from build123d import *

# Parameters (mm, degrees)
SKETCH1_W           = 145
SKETCH1_H           = 67
SKETCH1_R           = 1.5
BOSS_EXTRUDE1_DEPTH = 3.175
FILLET2_R           = 2


with BuildPart() as part:
    # Sketch1 → Boss-Extrude1 (new body)
    with BuildSketch(Plane.XY):
        Rectangle(SKETCH1_W, SKETCH1_H)
        with Locations((-35, 23.5)):
            Circle(SKETCH1_R, mode=Mode.SUBTRACT)
        with Locations((35, 23.5)):
            Circle(SKETCH1_R, mode=Mode.SUBTRACT)
        with Locations((35, -23.5)):
            Circle(SKETCH1_R, mode=Mode.SUBTRACT)
        with Locations((-35, -23.5)):
            Circle(SKETCH1_R, mode=Mode.SUBTRACT)
        with Locations((-27.5, 15)):
            Circle(SKETCH1_R, mode=Mode.SUBTRACT)
        with Locations((27.5, 15)):
            Circle(SKETCH1_R, mode=Mode.SUBTRACT)
        with Locations((27.5, -15)):
            Circle(SKETCH1_R, mode=Mode.SUBTRACT)
        with Locations((-27.5, -15)):
            Circle(SKETCH1_R, mode=Mode.SUBTRACT)
        with Locations((-69, 30)):
            Circle(SKETCH1_R, mode=Mode.SUBTRACT)
        with Locations((-50, 30)):
            Circle(SKETCH1_R, mode=Mode.SUBTRACT)
        with Locations((-50, -30)):
            Circle(SKETCH1_R, mode=Mode.SUBTRACT)
        with Locations((-69, -30)):
            Circle(SKETCH1_R, mode=Mode.SUBTRACT)
        with Locations((50, -30)):
            Circle(SKETCH1_R, mode=Mode.SUBTRACT)
        with Locations((69, -30)):
            Circle(SKETCH1_R, mode=Mode.SUBTRACT)
        with Locations((50, 30)):
            Circle(SKETCH1_R, mode=Mode.SUBTRACT)
        with Locations((69, 30)):
            Circle(SKETCH1_R, mode=Mode.SUBTRACT)
        Polygon((15.862719753, 0), (7.931359877, 13.737518279), (-7.931359877, 13.737518279), (-15.862719753, 0), (-7.931359877, -13.737518279), (7.931359877, -13.737518279), align=None, mode=Mode.SUBTRACT)
    extrude(amount=BOSS_EXTRUDE1_DEPTH)

    # Fillet2
    fillet2_edges = [part.edges().sort_by_distance(p)[0] for p in [
        (-72.5, 33.5, 1.5875),
        (72.5, 33.5, 1.5875),
        (72.5, -33.5, 1.5875),
        (-72.5, -33.5, 1.5875),
    ]]
    fillet(fillet2_edges, radius=FILLET2_R)


solid = part.part
The listing builds one solid part. Answer for the finished solid, in the listing's coordinates (mm). A direction names the side the tool comes from. Give positions to 0.01 mm unless a question says otherwise; leave off trailing zeros. Write each loop counter-clockwise with the first axis right and the second up, starting at its lowest first coordinate (ties: lowest second). Pieces come first, ordered by that corner, then holes. Notation, with made-up numbers: (88.5, 87.25) -> (127.5, 87.25) arc R12 cw to (127.5, 106.25) -> close; hole circle Ø7 at (-27.75, 68.5). An arc over 180 degrees is marked (long way). One line per question, with ' | ' between items. Start each with the question number.
1. For faces 4 (the flat face through (0, -13.738, 2)), 5 (the flat face through (72.5, 0, 2)), determine the directions among +Z, -Z, +X, -X, +Y, -Y from which every point of the face is accessible in a straight line to the end or side of a thin tool.
2. Section C-C (y = 30) is taken. Determine the outline of the cut face in (x, z) (3 decimals), plus the area to 3 significant figures.
3. Section D-D (y = -23.5) is taken. Determine the outline of the cut face in (x, z) (3 decimals).
4. Section B-B (z = 2.15) is taken. State how many separate pieces and enclosed holes the cut face has, plus the area to 3 significant figures.
5. Find the intervals of material crossed by probe 1 along Y at (x, z) = (69, 1.35); probe 2 along Y at (x, z) = (-35, 1.9); probe 3 along Y at (x, z) = (0.5, 1.2), in increasing order.
6. Given pin 1 Ø1.8 at (x, y) = (-35, -23.5) entering from -Z, flat-ended and moving along its own axis, determine where the tip first touches the part or whether it passes through.
7. Section A-A (x = 50) is taken. Determine the outline of the cut face in (y, z) (3 decimals).
8. For a pull along Y with two mould halves and no side action, classify faces 1 (the flat face through (-1, -33.5, 2)), 2 (the flat face through (-72.5, 0, 2)), 3 (the flat face through (-11.953, -6.773, 1.565)) as pulls with the +Y half, pulls with the -Y half, needs draft (parallel to the pull), parting line crosses it, or undercut.
Response values:
1) face 4: +Z, -Z | face 5: +Z, -Z, +X, +Y, -Y
2) outline: (-72.5, 0) -> (-70.5, 0) -> (-70.5, 3.175) -> (-72.5, 3.175) -> close; (-67.5, 0) -> (-51.5, 0) -> (-51.5, 3.175) -> (-67.5, 3.175) -> close; (-48.5, 0) -> (48.5, 0) -> (48.5, 3.175) -> (-48.5, 3.175) -> close; (51.5, 0) -> (67.5, 0) -> (67.5, 3.175) -> (51.5, 3.175) -> close; (70.5, 0) -> (72.5, 0) -> (72.5, 3.175) -> (70.5, 3.175) -> close | area: 422 mm2
3) outline: (-72.5, 0) -> (-36.5, 0) -> (-36.5, 3.175) -> (-72.5, 3.175) -> close; (-33.5, 0) -> (33.5, 0) -> (33.5, 3.175) -> (-33.5, 3.175) -> close; (36.5, 0) -> (72.5, 0) -> (72.5, 3.175) -> (36.5, 3.175) -> close
4) separate pieces: 1 | enclosed holes: 17 | area: 8,940 mm2
5) probe 1: -33.5 to -31.5, -28.5 to 28.5, 31.5 to 33.5 | probe 2: -33.5 to -25, -22 to 22, 25 to 33.5 | probe 3: -33.5 to -13.74, 13.74 to 33.5
6) pin 1: through
7) outline: (-33.5, 0) -> (-31.5, 0) -> (-31.5, 3.175) -> (-33.5, 3.175) -> close; (-28.5, 0) -> (28.5, 0) -> (28.5, 3.175) -> (-28.5, 3.175) -> close; (31.5, 0) -> (33.5, 0) -> (33.5, 3.175) -> (31.5, 3.175) -> close
8) face 1: pulls with the -Y half | face 2: needs draft | face 3: undercut
